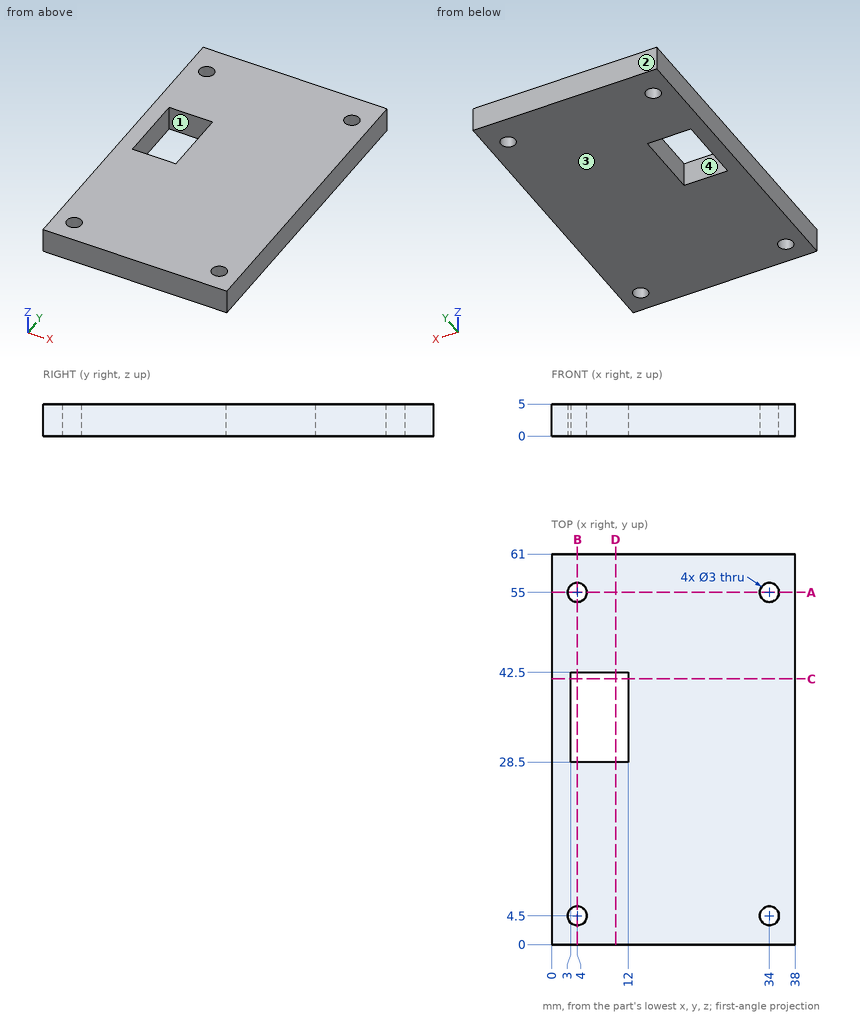
Could you check a few things on this drawing? It's one solid part, dimensions in mm from its lowest x, y, z. Coordinates: 2 decimals unless noted, no trailing zeros. Order: outer loops, then holes, each group sorted by start corner. A loop starts at its lowest first (then second) coordinate and runs counter-clockwise, first axis right, second up. Notation, with made-up numbers: M -30,70 L 22,70 A13 ccw 22,86 Z; hole C 6.5,31 d11. An arc over 180 degrees is marked long. Use a Markdown table: item, result. Add a question column.
Q1. I'm going to push a flat-ended pin straight in: pin 1 (1.8 mm diameter, centred on x = 34, y = 55, fed in from -Z). Where does the tip first touch, or does it pass through?
Q2. I want a section at B-B on x = 4. List the corners of the cut face in (y, z) for me.
Q3. We'd pull the mould along Y, two halves only. Please class the marked faces 1, 2, 3 and 4: pulls with the +Y half, pulls with the -Y half, needs draft (parallel to the pull), parting line crosses it, or undercut.
Q4. I want a section at C-C on y = 41.5. List the corners of the cut face in (x, z) for me, then the cut area to 3 significant figures.
Q5. I want a section at D-D on x = 10. List the corners of the cut face in (y, z) for me.
Q6. I want a section at A-A on y = 55. List the corners of the cut face in (x, z) for me.
Q7. If I drill on L1, parallel to X at y = 4.5, z = 2.35; L2, parallel to Y at x = 4, z = 3.75; L3, parallel to Y at x = 34, z = 3.35, over which ranges is the centre line in solid material (lowest first)?
Checked values:
| question | item | result |
|---|---|---|
| 1 | pin 1 | through |
| 2 | outline | M 0,0 L 3,0 L 3,5 L 0,5 Z; M 6,0 L 28.5,0 L 28.5,5 L 6,5 Z; M 42.5,0 L 53.5,0 L 53.5,5 L 42.5,5 Z; M 56.5,0 L 61,0 L 61,5 L 56.5,5 Z |
| 3 | face 1 | undercut |
| 3 | face 2 | pulls with the +Y half |
| 3 | face 3 | needs draft |
| 3 | face 4 | undercut |
| 4 | outline | M 0,0 L 3,0 L 3,5 L 0,5 Z; M 12,0 L 38,0 L 38,5 L 12,5 Z |
| 4 | area | 145 mm² |
| 5 | outline | M 0,0 L 28.5,0 L 28.5,5 L 0,5 Z; M 42.5,0 L 61,0 L 61,5 L 42.5,5 Z |
| 6 | outline | M 0,0 L 2.5,0 L 2.5,5 L 0,5 Z; M 5.5,0 L 32.5,0 L 32.5,5 L 5.5,5 Z; M 35.5,0 L 38,0 L 38,5 L 35.5,5 Z |
| 7 | L1 | 0 to 2.5, 5.5 to 32.5, 35.5 to 38 |
| 7 | L2 | 0 to 3, 6 to 28.5, 42.5 to 53.5, 56.5 to 61 |
| 7 | L3 | 0 to 3, 6 to 53.5, 56.5 to 61 |
